Verification items for the finished model (mm, model axes). Face numbers are marked on the shaded views. A direction names the side the tool comes from. Coordinates: 2 decimals unless noted, no trailing zeros. Order: outer loops, then holes, each group sorted by start corner. A loop starts at its lowest first (then second) coordinate and runs counter-clockwise, first axis right, second up.
Q1. Thickness scan on line 1 (X direction, y = 3.15, z = 0); line 2 (X direction, y = -0.75, z = 0); line 3 (Y direction, x = 0.25, z = 1.25). Record the ranges inside material, lowest first.
Q2. Depth check by flat-ended pin: P1, Ø1.5, axis at y = 9, z = 4.5, coming from the +X side; P2, Ø6, axis at x = 0, z = 0, coming from the -Y side; P3, Ø1, axis at y = 8.5, z = 1, coming from the +X side; P4, Ø5, axis at y = 3.5, z = 3.5, coming from the -X side. Enter the tip coordinate at first touch or a pass-through.
Q3. Set-up check for the marked faces 1, 2 and 3: record each of +Z, -Z, +X, -X, +Y, -Y from which the full face is reachable in a straight line by a thin tool's end or side.
Q4. Cross-section at C-C, the plane x = 0. Record the boundary of the cut face in (y, z).
Q5. Cross-section at D-D, the plane y = 2.5. Record the boundary of the cut face in (x, z).
Q6. Draft check along X on the marked faces 4, 5 and 6. Enter one of: pulls with the +X half, pulls with the -X half, needs draft (parallel to the pull), parting line crosses it, or undercut.
Q7. Cross-section at B-B, the plane z = 0. Record the boundary of the cut face in (x, y).
Q8. Cross-section at A-A, the plane y = 8.75. Record the boundary of the cut face in (x, z).
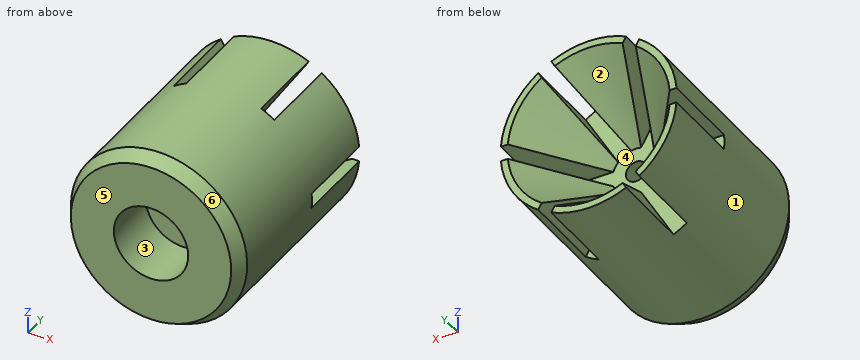
from build123d import *

# Parameters (mm, degrees)
CHAMFER1_SIZE      = 1
CHAMFER1_SIZE2     = 0.577350269
SKETCH2_W          = 6.4
SKETCH2_H          = 5.926814228
CUT_EXTRUDE1_DEPTH = 0.55
CIRPATTERN1_COUNT  = 6


with BuildPart() as part:
    # Sketch1 → Revolve1 (revolve)
    with BuildSketch(Plane.XY, mode=Mode.PRIVATE) as revolve1_sk:
        Polygon((0, 0), (0, 0.5), (0.75, 0.5), (0.75, 5.073185772), (1.75, 5.073185772), (5.9, 11), (6.4, 11), (6.4, -4), (2.7, -4), (2.7, 0), align=None)
    revolve(revolve1_sk.sketch.rotate(Axis((0, 0, 0), (0, 1, 0)), 90), axis=Axis((0, 0, 0), (0, 1, 0)))

    # Chamfer1
    chamfer1_edges = [part.edges().sort_by_distance(p)[0] for p in [
        (0, -4, 6.4),
    ]]
    chamfer1_side = [part.faces().sort_by_distance(p)[0] for p in [
        (0, 3.5, 6.4),
    ]]
    chamfer(chamfer1_edges, length=CHAMFER1_SIZE, length2=CHAMFER1_SIZE2, reference=chamfer1_side[0])

    # Sketch2 → Cut-Extrude1 (cut, symmetric)
    with BuildSketch(Plane(origin=(0, 0, 0), x_dir=(-1, 0, 0), z_dir=(0, 0, -1))):
        with Locations((-3.2, 8.036592886)):
            Rectangle(SKETCH2_W, SKETCH2_H)
    cut_extrude1 = extrude(amount=CUT_EXTRUDE1_DEPTH, both=True, mode=Mode.SUBTRACT)

    # CirPattern1: Cut-Extrude1 ×6 about axis
    cirpattern1_axis = Axis((0, 0, 0), (0, 1, 0))
    for i in range(1, CIRPATTERN1_COUNT):
        add(cut_extrude1.rotate(cirpattern1_axis, i * 360 / CIRPATTERN1_COUNT), mode=Mode.SUBTRACT)


solid = part.part
Check values:
1. line 1: x = -6.4 to -0.75, 0.75 to 6.4
1. line 2: x = -6.4 to -2.7, 2.7 to 6.4
1. line 3: y = 0 to 5.07
2. P1: stops at x = 5.19
2. P2: stops at y = -4
2. P3: stops at x = 6.38
2. P4: stops at x = -6.32
3. face 1: +Y, -Y
3. face 2: +Y
3. face 3: -Y
4. outline: (-4, -5.82) - (-3, -6.4) - (11, -6.4) - (11, -5.9) - (5.07, -1.75) - (5.07, -0.75) - (0.5, -0.75) - (0.5, 0.75) - (5.07, 0.75) - (5.07, 1.75) - (11, 5.9) - (11, 6.4) - (-3, 6.4) - (-4, 5.82) - (-4, 2.7) - (0, 2.7) - (0, -2.7) - (-4, -2.7) - close
5. outline: circle Ø12.8 at (0, 0); hole circle Ø1.5 at (0, 0)
6. face 4: undercut
6. face 5: needs draft
6. face 6: parting line crosses it
7. outline: (-6.4, -3) - (-5.82, -4) - (-2.7, -4) - (-2.7, 0) - (2.7, 0) - (2.7, -4) - (5.82, -4) - (6.4, -3) - (6.4, 5.07) - (0.75, 5.07) - (0.75, 0.5) - (-0.75, 0.5) - (-0.75, 5.07) - (-6.4, 5.07) - close
8. outline: (-6.38, -0.55) arc R6.4 ccw to (-3.66, -5.25) - (-2.62, -3.44) arc R4.32 cw to (-4.29, -0.55) - close; (-6.38, 0.55) - (-4.29, 0.55) arc R4.32 cw to (-2.62, 3.44) - (-3.66, 5.25) arc R6.4 ccw to start; (-2.71, -5.8) arc R6.4 ccw to (2.71, -5.8) - (1.67, -3.99) arc R4.32 cw to (-1.67, -3.99) - close; (-2.71, 5.8) - (-1.67, 3.99) arc R4.32 cw to (1.67, 3.99) - (2.71, 5.8) arc R6.4 ccw to start; (2.62, -3.44) - (3.66, -5.25) arc R6.4 ccw to (6.38, -0.55) - (4.29, -0.55) arc R4.32 cw to start; (2.62, 3.44) arc R4.32 cw to (4.29, 0.55) - (6.38, 0.55) arc R6.4 ccw to (3.66, 5.25) - close
